Geometry check sheet. Reference: the model listing, model coordinates, mm. Round coordinates to 2 decimals unless told otherwise and drop trailing zeros. Loops run counter-clockwise (first coordinate to the right, second up) from the corner with the lowest first, then second, coordinate; pieces in that order, holes last.
```python
from build123d import *

# Parameters (mm, degrees)
SKETCH6_R           = 6.35
BOSS_EXTRUDE1_DEPTH = 127
LOFT6_START         = -6.35
LOFT6_DEPTH         = 12.6999999
LOFT6_START_2       = -3.8100001
LOFT6_2_DEPTH       = 7.6200001
LOFT6_START_3       = -10
LOFT6_3_DEPTH       = 20


with BuildPart() as part:
    # Sketch3 → Revolve2 (revolve)
    with BuildSketch(Plane(origin=(0, 0, 0), x_dir=(0, 1, 0), z_dir=(0, 0, 1)), mode=Mode.PRIVATE) as revolve2_sk:
        with BuildLine():
            ThreePointArc((19.05, 57.15), (10.450520825, 38.1), (19.05, 19.05))
            Line((19.05, 19.05), (19.05, 0))
            Line((19.05, 0), (0, 0))
            Line((0, 0), (0, 165.1))
            ThreePointArc((0, 165.1), (13.470384182, 159.520384182), (19.05, 146.05))
            Line((19.05, 146.05), (19.05, 57.15))
        make_face()
    revolve(revolve2_sk.sketch.rotate(Axis((0, 0, 0), (-1, 0, 0)), 90), axis=Axis((0, 0, 0), (-1, 0, 0)))

    # Sketch6 → Boss-Extrude1 (add)
    with BuildSketch(Plane.YZ):
        with Locations(Location((0, 0, 0), (0, 0, 270))):
            Circle(SKETCH6_R)
    extrude(amount=BOSS_EXTRUDE1_DEPTH)

    # Sketch7 for Loft5 → Loft5 section 0
    with BuildSketch(Plane(origin=(127, 0, 0), x_dir=(0, 0, -1), z_dir=(1, 0, 0))):
        with BuildLine():
            # circular arc as an exact rational Bezier (weights 1, cos(half-angle), 1)
            Bezier((-5.836570941, 2.501387546), (0, 16.120053073), (5.836570941, 2.501387546), weights=[1, 0.393919299, 1])
            Bezier((5.836570941, 2.501387546), (6.908594174, 0), (5.836570941, -2.501387546), weights=[1, 0.91914503, 1])
            Bezier((5.836570941, -2.501387546), (0, -16.120053073), (-5.836570941, -2.501387546), weights=[1, 0.393919299, 1])
            Bezier((-5.836570941, -2.501387546), (-6.908594174, 0), (-5.836570941, 2.501387546), weights=[1, 0.91914503, 1])
        make_face()
    # Sketch4 → Loft5 section 1
    with BuildSketch(Plane(origin=(152.4, 0, 0), x_dir=(0, 0, -1), z_dir=(1, 0, 0))):
        with BuildLine():
            Line((-8.89, 3.81), (8.89, 3.81))
            Line((8.89, 3.81), (8.89, -3.81))
            Line((8.89, -3.81), (-8.89, -3.81))
            Line((-8.89, -3.81), (-8.89, 3.81))
        make_face()
    loft()

    # Loft6: read off the stored shape, not the designer's step
    # Loft6 outline → Loft6 (add)
    with BuildSketch(Plane.XY.offset(LOFT6_START)):
        with BuildLine():
            Line((177.8, -1.27), (177.8, 1.27))
            add(Edge.make_bspline(
                [(177.8, 1.27), (169.375457091, 2.54), (160.950914181, 3.81), (152.4, 3.81)],
                knots=[0, 0, 0, 0, 1, 1, 1, 1], degree=3))
            Line((152.4, 3.81), (152.4, -3.81))
            add(Edge.make_bspline(
                [(177.8, -1.27), (169.375457091, -2.54), (160.950914181, -3.81), (152.4, -3.81)],
                knots=[0, 0, 0, 0, 1, 1, 1, 1], degree=3))
        make_face()
    extrude(amount=LOFT6_DEPTH)

    # Loft6 2 outline → Loft6 2 (add)
    with BuildSketch(Plane(origin=(0, 0, 0), x_dir=(1, 0, 0), z_dir=(0, 1, 0)).offset(LOFT6_START_2)):
        with BuildLine():
            Line((152.4, 6.35), (177.8, 6.35))
            add(Edge.make_bspline(
                [(177.8, 6.35), (169.375457091, 7.62), (160.950914181, 8.89), (152.4, 8.89)],
                knots=[0, 0, 0, 0, 1, 1, 1, 1], degree=3))
            Line((152.4, 8.89), (152.4, 6.35))
        make_face()
        with BuildLine():
            add(Edge.make_bspline(
                [(177.8, -6.35), (169.375457091, -7.62), (160.950914181, -8.89), (152.4, -8.89)],
                knots=[0, 0, 0, 0, 1, 1, 1, 1], degree=3))
            Line((177.8, -6.35), (152.4, -6.3499999))
            Line((152.4, -6.3499999), (152.4, -8.89))
        make_face()
    extrude(amount=LOFT6_2_DEPTH)

    # Loft6 3 outline → Loft6 3 (cut)
    with BuildSketch(Plane.XY.offset(LOFT6_START_3)):
        with BuildLine():
            add(Edge.make_bspline(
                [(177.8, 1.27), (169.375457091, 2.54), (160.950914181, 3.81), (152.4, 3.81)],
                knots=[0, 0, 0, 0, 1, 1, 1, 1], degree=3))
            Line((177.8, 1.27), (177.8, 3.81))
            Line((177.8, 3.81), (152.4, 3.81))
        make_face()
        with BuildLine():
            add(Edge.make_bspline(
                [(177.8, -1.27), (169.375457091, -2.54), (160.950914181, -3.81), (152.4, -3.81)],
                knots=[0, 0, 0, 0, 1, 1, 1, 1], degree=3))
            Line((152.4, -3.81), (177.8, -3.8100001))
            Line((177.8, -3.8100001), (177.8, -1.27))
        make_face()
    extrude(amount=LOFT6_3_DEPTH, mode=Mode.SUBTRACT)


solid = part.part
```
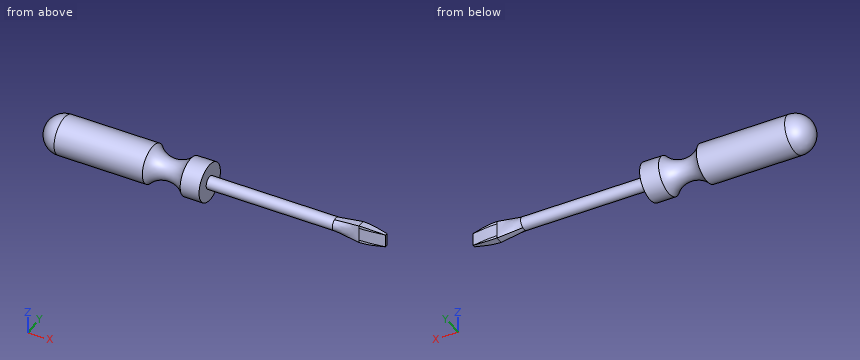
1) Sectioned sample at B-B, the plane x = 55. Record the cut outline in (y, z).
Report:
outline: circle Ø12.7 at (0, 0)
2) Sectioned sample at A-A, the plane x = -89.5. Record the cut outline in (y, z), then the cut area to 3 significant figures.
Report:
outline: circle Ø38.1 at (0, 0)
area: 1,140 mm2
3) Gauge pin test, flat ends, axial feed: pin 1 (1 mm diameter, centred on y = -2, z = 9.5, fed in from -X); pin 2 (10 mm diameter, centred on x = -123.5, z = 8.5, fed in from +Y); pin 3 (1.5 mm diameter, centred on x = 29.5, z = 6, fed in from +Y); pin 4 (10 mm diameter, centred on x = 64.5, y = -15, fed in from -Z). Record the tip position at first contact, or that the pin passes through.
Report:
pin 1: stops at x = -162.73
pin 2: stops at y = 18.73
pin 3: stops at y = 3.57
pin 4: passes through
4) Scan lines: line 1 along X through (y, z) = (-2.5, -17); line 2 along Y through (x, z) = (46, 0.5); line 3 along X through (y, z) = (1, -15.5). Record each from-to range of solid material in increasing order.
Report:
line 1: x = -154.28 to -55.32, -20.88 to 0
line 2: y = -6.33 to 6.33
line 3: x = -157.08 to -53.34, -22.86 to 0
